The drawing under review shows one solid part. Ordinate dimensions are in mm from its lowest x, y, z. A direction names the side the tool comes from. Coordinates: 2 decimals unless noted, no trailing zeros. Order: outer loops, then holes, each group sorted by start corner. A loop starts at its lowest first (then second) coordinate and runs counter-clockwise, first axis right, second up.
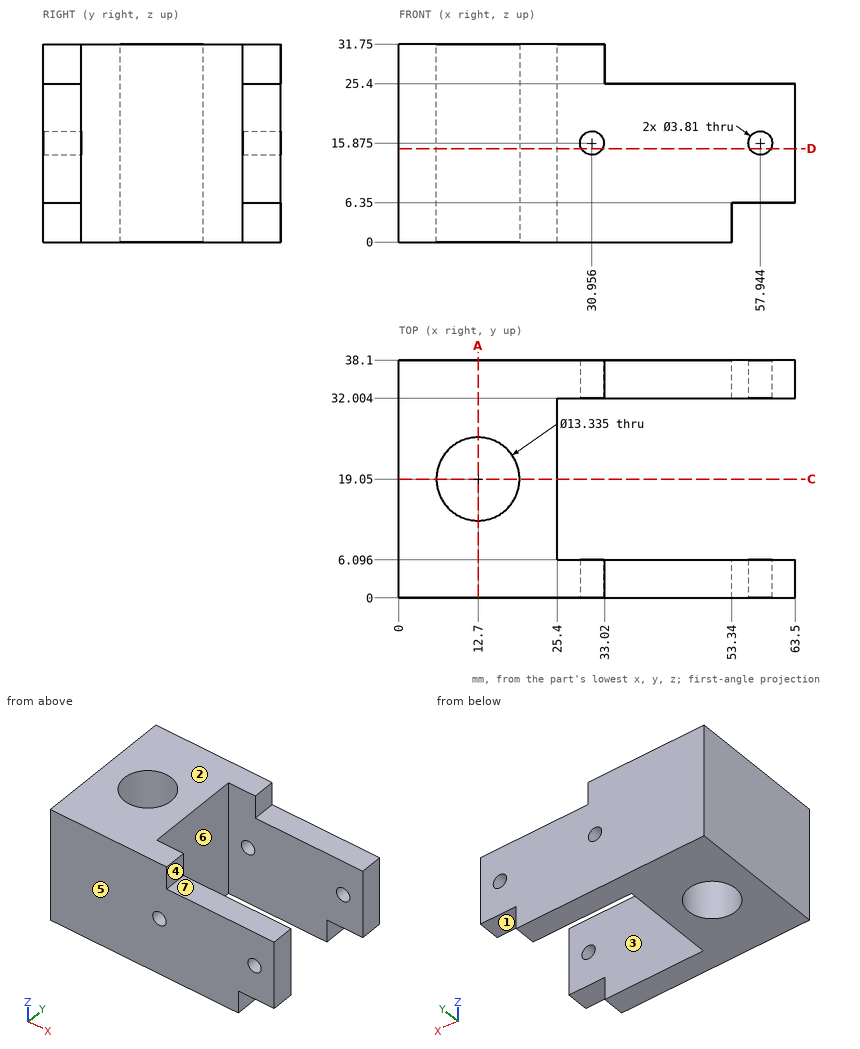
(1) The part is to be moulded in two halves that separate along Y. For the marked faces 5, 6 and 7, say which applies: +Y half, -Y half, draft (parallel to the pull), parting line (faces both ways), or undercut.
(2) Consider section C-C (y = 19.05). Give the boundary of the cut face in (x, z).
(3) Insertion check: pin 1 Ø3 at (x, y) = (48.5, 2.5) entering from +Z; pin 2 Ø3 at (y, z) = (3.5, 28.5) entering from +X; pin 3 Ø3 at (x, y) = (59, 4) entering from -Z. Each pin has a flat end and moves straight along its axis. Give the tip position at first contact, or say it passes through.
(4) Tool access review of the marked faces 1, 2, 3 and 4: name each direction out of +Z, -Z, +X, -X, +Y, -Y from which nothing blocks a thin tool from reaching the whole face with its end or side.
(5) Wall thickness on line 1 (Y direction, x = 42.5, z = 14); line 2 (Y direction, x = 13, z = 22.5); line 3 (X direction, y = 12, z = 2.5): over which ranges is each line inside the solid? List them lowest first.
(6) Consider section D-D (z = 15). Give the number of separate pieces and of enclosed holes in the cut face, then the cut area to 3 significant figures.
(7) Consider section A-A (x = 12.7). Give the boundary of the cut face in (y, z).
Findings:
1. face 5: -Y half
1. face 6: undercut
1. face 7: draft
2. outline: (0, 0) - (6.03, 0) - (6.03, 31.75) - (0, 31.75) - close; (19.37, 0) - (25.4, 0) - (25.4, 31.75) - (19.37, 31.75) - close
3. pin 1: stops at z = 25.4
3. pin 2: stops at x = 33.02
3. pin 3: stops at z = 6.35
4. face 1: -Z, +X, +Y, -Y
4. face 2: +Z, +X, -X, +Y, -Y
4. face 3: +Z, -Z, +X
4. face 4: +Z, +X, +Y, -Y
5. line 1: y = 0 to 6.1, 32 to 38.1
5. line 2: y = 0 to 12.39, 25.71 to 38.1
5. line 3: x = 0 to 25.4
6. separate pieces: 5
6. enclosed holes: 1
6. area: 1,210 mm2
7. outline: (0, 0) - (12.38, 0) - (12.38, 31.75) - (0, 31.75) - close; (25.72, 0) - (38.1, 0) - (38.1, 31.75) - (25.72, 31.75) - close
